Read the model definition and answer for the solid it produces. Units are mm, in the model's axes. Face numbers are marked on the shaded views. Coordinates: 2 decimals unless noted, no trailing zeros. Loops run counter-clockwise (first coordinate to the right, second up) from the corner with the lowest first, then second, coordinate; pieces in that order, holes last.
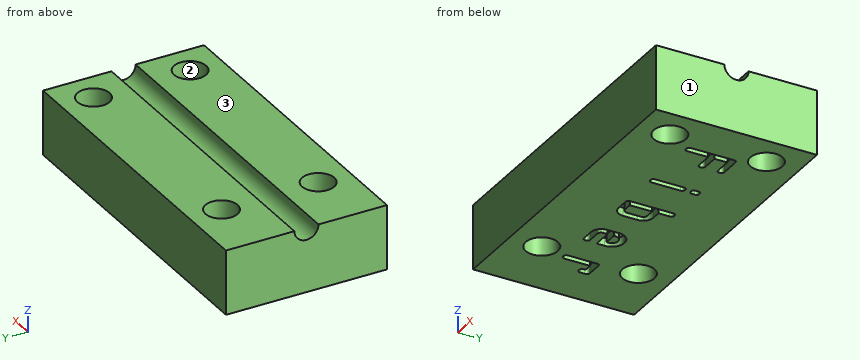
Autodesk Inventor part; units mm, degrees
ref_plane "YZ Plane" through (0, 0, 0) normal (1, 0, 0) x (0, 1, 0)
ref_plane "XZ Plane" through (0, 0, 0) normal (0, 1, 0) x (-1, 0, 0)
ref_plane "XY Plane" through (0, 0, 0) normal (0, 0, 1) x (1, 0, 0)
sketch "Sketch3" plane through (0, 0, 0) normal (0, 0, 1) x (1, 0, 0)
  line L0 (-10, 5) -> (10, 5)
  line L1 (10, 5) -> (10, -5)
  line L2 (10, -5) -> (-10, -5)
  line L3 (-10, -5) -> (-10, 5)
  line L4 (-10, 5) -> (10, -5) construction
  line L5 (10, 5) -> (-10, -5) construction
  point P0 (0, 0)
  dimension "d5" = 20
  dimension "d6" = 10
extrude "Extrusion2" add sketch "Sketch3" along normal blind 4
sketch "Sketch4" plane through (10, -5, 0) normal (1, 0, 0) x (0, 0, -1)
  circle A0 centre (-4, 5) radius 0.75
  point P0 (0, 5)
  dimension "d10" = 1.5
extrude "Extrusion3" cut sketch "Sketch4" against normal through all
sketch "Sketch5" plane through (0, 0, 4) normal (0, 0, 1) x (1, 0, 0)
  circle A0 centre (8, 3) radius 1
  circle A1 centre (8, -3) radius 1
  circle A2 centre (-6, 3) radius 1
  circle A3 centre (-6, -3) radius 1
  point P0 (0, 0)
  dimension "d17" = 2
  dimension "d16" = 2
  dimension "d15" = 2
  dimension "d14" = 2
extrude "Extrusion4" cut sketch "Sketch5" against normal through all
sketch "Sketch6" plane through (0, 0, 0) normal (0, 0, -1) x (-1, 0, 0)
  line L0 (-8.1739, 1.5824) -> (1.6987, 1.5824) construction
  line L1 (1.6987, 1.5824) -> (1.6987, -1.5298) construction
  line L2 (1.6987, -1.5298) -> (-8.1739, -1.5298) construction
  line L3 (-8.1739, -1.5298) -> (-8.1739, 1.5824) construction
  line L4 (-7.2861, -1.2743) -> (-7.2861, 1.3892)
  spline S0 degree 2 poles (-7.2861, 1.3892) (-7.2861, 1.5824) (-7.09, 1.5824) knots 0 0 0 1 1 1
  line L5 (-7.09, 1.5824) -> (-5.9053, 1.5824)
  spline S1 degree 2 poles (-5.9053, 1.5824) (-5.7093, 1.5824) (-5.7093, 1.3892) knots 0 0 0 1 1 1
  spline S2 degree 2 poles (-5.7093, 1.3892) (-5.7093, 1.1931) (-5.9053, 1.1931) knots 0 0 0 1 1 1
  line L6 (-5.9053, 1.1931) -> (-6.894, 1.1931)
  line L7 (-6.894, 1.1931) -> (-6.894, 0.3977)
  line L8 (-6.894, 0.3977) -> (-5.9053, 0.3977)
  spline S3 degree 2 poles (-5.9053, 0.3977) (-5.7093, 0.3977) (-5.7093, 0.2045) knots 0 0 0 1 1 1
  spline S4 degree 2 poles (-5.7093, 0.2045) (-5.7093, 0.0084) (-5.9053, 0.0084) knots 0 0 0 1 1 1
  line L9 (-5.9053, 0.0084) -> (-6.894, 0.0084)
  line L10 (-6.894, 0.0084) -> (-6.894, -1.2743)
  spline S5 degree 2 poles (-6.894, -1.2743) (-6.894, -1.4704) (-7.09, -1.4704) knots 0 0 0 1 1 1
  spline S6 degree 2 poles (-7.09, -1.4704) (-7.2861, -1.4704) (-7.2861, -1.2743) knots 0 0 0 1 1 1
  spline S7 degree 2 poles (-3.3734, 0.5014) (-3.3734, 0.6918) (-3.1774, 0.6918) knots 0 0 0 1 1 1
  spline S8 degree 2 poles (-3.1774, 0.6918) (-2.9813, 0.6918) (-2.9813, 0.5014) knots 0 0 0 1 1 1
  line L11 (-2.9813, 0.5014) -> (-2.9813, -1.2743)
  spline S9 degree 2 poles (-2.9813, -1.2743) (-2.9813, -1.4704) (-3.1774, -1.4704) knots 0 0 0 1 1 1
  spline S10 degree 2 poles (-3.1774, -1.4704) (-3.3734, -1.4704) (-3.3734, -1.2743) knots 0 0 0 1 1 1
  line L12 (-3.3734, -1.2743) -> (-3.3734, 0.5014)
  line L13 (-3.3734, 1.2379) -> (-3.3734, 1.3864)
  spline S11 degree 2 poles (-3.3734, 1.3864) (-3.3734, 1.5796) (-3.1774, 1.5796) knots 0 0 0 1 1 1
  spline S12 degree 2 poles (-3.1774, 1.5796) (-2.9813, 1.5796) (-2.9813, 1.3864) knots 0 0 0 1 1 1
  line L14 (-2.9813, 1.3864) -> (-2.9813, 1.2379)
  spline S13 degree 2 poles (-2.9813, 1.2379) (-2.9813, 1.0447) (-3.1774, 1.0447) knots 0 0 0 1 1 1
  spline S14 degree 2 poles (-3.1774, 1.0447) (-3.3734, 1.0447) (-3.3734, 1.2379) knots 0 0 0 1 1 1
  line L15 (0.9313, 0.0588) -> (0.9313, -0.8318)
  spline S15 degree 2 poles (0.9313, -0.8318) (0.9313, -1.1007) (0.5616, -1.4704) (0.2927, -1.4704) knots 0 0 0 1 2 2 2
  line L16 (0.2927, -1.4704) -> (-0.4467, -1.4704)
  spline S16 degree 2 poles (-0.4467, -1.4704) (-0.6427, -1.4704) (-0.6427, -1.2743) knots 0 0 0 1 1 1
  line L17 (-0.6427, -1.2743) -> (-0.6427, 1.3864)
  spline S17 degree 2 poles (-0.6427, 1.3864) (-0.6427, 1.5796) (-0.4467, 1.5796) knots 0 0 0 1 1 1
  spline S18 degree 2 poles (-0.4467, 1.5796) (-0.2506, 1.5796) (-0.2506, 1.3864) knots 0 0 0 1 1 1
  line L18 (-0.2506, 1.3864) -> (-0.2506, 0.6946)
  line L19 (-0.2506, 0.6946) -> (0.2927, 0.6946)
  spline S19 degree 2 poles (0.2927, 0.6946) (0.6652, 0.6946) (0.8473, 0.3781) knots 0 0 0 1 1 1
  spline S20 degree 2 poles (0.8473, 0.3781) (0.9313, 0.2297) (0.9313, 0.0588) knots 0 0 0 1 1 1
  line L20 (0.2927, 0.3053) -> (-0.2506, 0.3053)
  line L21 (-0.2506, 0.3053) -> (-0.2506, -1.0811)
  line L22 (-0.2506, -1.0811) -> (0.2927, -1.0811)
  spline S21 degree 2 poles (0.2927, -1.0811) (0.3935, -1.0811) (0.5392, -0.9354) (0.5392, -0.829) knots 0 0 0 1 2 2 2
  line L23 (0.5392, -0.829) -> (0.5392, 0.056)
  spline S22 degree 2 poles (0.5392, 0.056) (0.5392, 0.1625) (0.3963, 0.3053) (0.2927, 0.3053) knots 0 0 0 1 2 2 2
  line L24 (3.071, -0.5825) -> (3.071, -0.829)
  spline S23 degree 2 poles (3.071, -0.829) (3.071, -0.9326) (3.2195, -1.0811) (3.3203, -1.0811) knots 0 0 0 1 2 2 2
  line L25 (3.3203, -1.0811) -> (4.0597, -1.0811)
  spline S24 degree 2 poles (4.0597, -1.0811) (4.2558, -1.0811) (4.2558, -1.2743) knots 0 0 0 1 1 1
  spline S25 degree 2 poles (4.2558, -1.2743) (4.2558, -1.4704) (4.0597, -1.4704) knots 0 0 0 1 1 1
  line L26 (4.0597, -1.4704) -> (3.3203, -1.4704)
  spline S26 degree 2 poles (3.3203, -1.4704) (3.0486, -1.4704) (2.6789, -1.1007) (2.6789, -0.8318) knots 0 0 0 1 2 2 2
  line L27 (2.6789, -0.8318) -> (2.6789, -0.0924)
  spline S27 degree 2 poles (2.6789, -0.0924) (2.6789, 0.2325) (3.1383, 0.6918) (3.4659, 0.6918) knots 0 0 0 1 2 2 2
  spline S28 degree 2 poles (3.4659, 0.6918) (3.7992, 0.6918) (4.2558, 0.2381) (4.2558, -0.0924) knots 0 0 0 1 2 2 2
  line L28 (4.2558, -0.0924) -> (4.2558, -0.5825)
  line L29 (4.2558, -0.5825) -> (3.071, -0.5825)
  spline S29 degree 2 poles (3.4659, 0.3053) (3.3035, 0.3053) (3.071, 0.0728) (3.071, -0.0896) knots 0 0 0 1 2 2 2
  line L30 (3.071, -0.0896) -> (3.071, -0.1932)
  line L31 (3.071, -0.1932) -> (3.8636, -0.1932)
  line L32 (3.8636, -0.1932) -> (3.8636, -0.0896)
  spline S30 degree 2 poles (3.8636, -0.0896) (3.8636, 0.0728) (3.6312, 0.3053) (3.4659, 0.3053) knots 0 0 0 1 2 2 2
  spline S31 degree 2 poles (6.149, 0.5014) (6.149, 0.6946) (6.3451, 0.6946) knots 0 0 0 1 1 1
  line L33 (6.3451, 0.6946) -> (7.2329, 0.6946)
  spline S32 degree 2 poles (7.2329, 0.6946) (7.429, 0.6946) (7.429, 0.5014) knots 0 0 0 1 1 1
  line L34 (7.429, 0.5014) -> (7.429, 0.2045)
  spline S33 degree 2 poles (7.429, 0.2045) (7.429, 0.0084) (7.2329, 0.0084) knots 0 0 0 1 1 1
  spline S34 degree 2 poles (7.2329, 0.0084) (7.0369, 0.0084) (7.0369, 0.2045) knots 0 0 0 1 1 1
  line L35 (7.0369, 0.2045) -> (7.0369, 0.3053)
  line L36 (7.0369, 0.3053) -> (6.5412, 0.3053)
  line L37 (6.5412, 0.3053) -> (6.5412, -1.2743)
  spline S35 degree 2 poles (6.5412, -1.2743) (6.5412, -1.4704) (6.3451, -1.4704) knots 0 0 0 1 1 1
  spline S36 degree 2 poles (6.3451, -1.4704) (6.149, -1.4704) (6.149, -1.2743) knots 0 0 0 1 1 1
  line L38 (6.149, -1.2743) -> (6.149, 0.5014)
  point P0 (0, 0)
extrude "Extrusion5" cut sketch "Sketch6" against normal blind 0.5
properties part number "fiber_top"
Item 1: Given pin 1 (1.3 mm diameter, centred on x = 6.5, y = 0.5, fed in from -Z), flat-ended and moving along its own axis, determine where the tip first touches the part or whether it passes through.
Numbers:
pin 1: stops at z = 0
Item 2: A cutting plane is placed at C-C on z = 1.6. Determine the outline of the cut face in (x, y).
Numbers:
outline: (-10, -5) - (10, -5) - (10, 5) - (-10, 5) - close; hole circle Ø2 at (-6, -3); hole circle Ø2 at (-6, 3); hole circle Ø2 at (8, -3); hole circle Ø2 at (8, 3)
Item 3: Find the intervals of material crossed by line 1 along Y through (x, z) = (8, 1.8); line 2 along Y through (x, z) = (-3.5, 0.2); line 3 along Y through (x, z) = (-6.75, 1.25), in increasing order.
Numbers:
line 1: y = -5 to -4, -2 to 2, 4 to 5
line 2: y = -5 to -1.47, -1.08 to -0.58, -0.19 to 0.3, 0.69 to 5
line 3: y = -5 to -3.66, -2.34 to 2.34, 3.66 to 5
Item 4: Determine the mould class of the marked faces 1, 2 and 3 for opening direction X: released by +X, released by -X, zero draft, split by the parting line, or undercut.
Numbers:
face 1: released by +X
face 2: undercut
face 3: zero draft
Item 5: A cutting plane is placed at A-A on x = 8. Determine the outline of the cut face in (y, z).
Numbers:
outline: (-5, 0) - (-4, 0) - (-4, 4) - (-5, 4) - close; (-2, 0) - (2, 0) - (2, 4) - (0.75, 4) arc R0.75 cw to (-0.75, 4) - (-2, 4) - close; (4, 0) - (5, 0) - (5, 4) - (4, 4) - close
Item 6: A cutting plane is placed at D-D on y = -3.25. Determine the outline of the cut face in (x, z).
Numbers:
outline: (-10, 0) - (-6.97, 0) - (-6.97, 4) - (-10, 4) - close; (-5.03, 0) - (7.03, 0) - (7.03, 4) - (-5.03, 4) - close; (8.97, 0) - (10, 0) - (10, 4) - (8.97, 4) - close
Item 7: A cutting plane is placed at B-B on y = 3. Determine the outline of the cut face in (x, z).
Numbers:
outline: (-10, 0) - (-7, 0) - (-7, 4) - (-10, 4) - close; (-5, 0) - (7, 0) - (7, 4) - (-5, 4) - close; (9, 0) - (10, 0) - (10, 4) - (9, 4) - close
